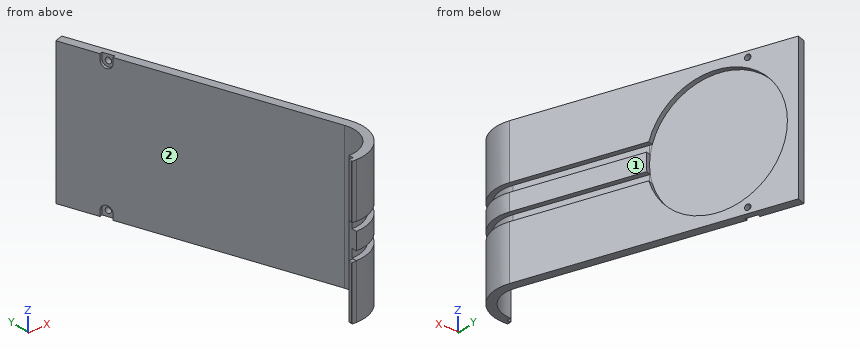
```python
from build123d import *

# Parameters (mm, degrees)
EXTRUDE_1_DEPTH        = 25
SKETCH_4_R             = 22
CUT_EXTRUDE_1_DEPTH    = 1.8
CUT_EXTRUDE_START      = 6
CUT_EXTRUDE_1_2_DEPTH  = 3
SKETCH_11_W            = 18.9
SKETCH_11_H            = 1.4
EXTRUDE_3_DEPTH        = 1.5
FILLET_1_R             = 0.25
SKETCH_12_R            = 1
CUT_EXTRUDE_2553_DEPTH = 99.437390504
CUT_EXTRUDE_1_3_DEPTH  = 1


with BuildPart() as part:
    # 草图2 → 整体拉伸-薄壁1 (new, symmetric)
    with BuildSketch(Plane.XY):
        with BuildLine():
            ThreePointArc((28.874192719, 5.049687275), (37.065713162, 9.313922912), (38.271118927, 18.469888708))
            Line((38.271118927, 18.469888708), (7.496652644, 103.022039918))
            Line((7.496652644, 103.022039918), (10.315730506, 104.048100348))
            Line((10.315730506, 104.048100348), (41.090196789, 19.495949138))
            ThreePointArc((41.090196789, 19.495949138), (39.523169295, 7.593193603), (28.874192719, 2.049687275))
            Line((28.874192719, 2.049687275), (28.874192719, 5.049687275))
        make_face()
    extrude(amount=EXTRUDE_1_DEPTH, both=True)

    # 草图4 → Cut-Extrude 1 (cut)
    with BuildSketch(Plane(origin=(42.549434126, 15.486727507, 0), x_dir=(0, 0, -1), z_dir=(0.9396926207859071, 0.3420201433256726, 0))):
        with Locations(Location((0, 68.845044478, 0), (0, 0, 90))):
            Circle(SKETCH_4_R)
    extrude(amount=-CUT_EXTRUDE_1_DEPTH, mode=Mode.SUBTRACT)

    # 草图3 → Cut-Extrude 1 2 (cut)
    with BuildSketch(Plane.XY.offset(CUT_EXTRUDE_START)):
        with BuildLine():
            ThreePointArc((28.874192719, 3.849687275), (38.048695615, 8.625631188), (39.398750072, 18.88031288))
            Line((39.398750072, 18.88031288), (24.836038582, 58.891033865))
            Line((24.836038582, 58.891033865), (23.809978152, 61.710111727))
            Line((23.809978152, 61.710111727), (25.50142487, 62.325747985))
            Line((25.50142487, 62.325747985), (26.5274853, 59.506670123))
            Line((26.5274853, 59.506670123), (41.090196789, 19.495949138))
            ThreePointArc((41.090196789, 19.495949138), (39.523169295, 7.593193603), (28.874192719, 2.049687275))
            Line((28.874192719, 2.049687275), (28.874192719, 3.849687275))
        make_face()
    cut_extrude_1_2 = extrude(amount=-CUT_EXTRUDE_1_2_DEPTH, mode=Mode.SUBTRACT)

    # 镜向1: Cut-Extrude 1 2 across plane
    add(cut_extrude_1_2.mirror(Plane.XY), mode=Mode.SUBTRACT)

    # 草图11 → 底部卡扣凸台-拉伸3 (add)
    with BuildSketch(Plane.ZY.offset(-28.874192719)):
        with Locations((-15.55, 2.749687275)):
            Rectangle(SKETCH_11_W, SKETCH_11_H)
        with Locations((15.55, 2.749687275)):
            Rectangle(SKETCH_11_W, SKETCH_11_H)
    extrude(amount=EXTRUDE_3_DEPTH)

    # 底部卡扣圆角1
    fillet_1_edges = [part.edges().sort_by_distance(p)[0] for p in [
        (27.374192719, 2.749687275, -25),
        (27.374192719, 2.049687275, -15.55),
        (27.374192719, 2.749687275, -6.1),
        (27.374192719, 3.449687275, -15.55),
        (27.374192719, 2.749687275, 6.1),
        (27.374192719, 2.049687275, 15.55),
        (27.374192719, 2.749687275, 25),
        (27.374192719, 3.449687275, 15.55),
    ]]
    fillet(fillet_1_edges, radius=FILLET_1_R)

    # 草图12 → Cut-Extrude 2553 (cut, through all)
    with BuildSketch(Plane(origin=(39.730356264, 14.460667077, 0), x_dir=(0, 0, 1), z_dir=(-0.9396926207859071, -0.3420201433256726, 0))):
        with Locations(Location((23, 78.482840932, 0), (0, 0, 270))):
            Circle(SKETCH_12_R)
        with Locations(Location((-23, 78.482840932, 0), (0, 0, 270))):
            Circle(SKETCH_12_R)
    extrude(amount=-CUT_EXTRUDE_2553_DEPTH, mode=Mode.SUBTRACT)

    # 草图13 → Cut-Extrude 1 3 (cut)
    with BuildSketch(Plane(origin=(39.730356264, 14.460667077, 0), x_dir=(0, 0, 1), z_dir=(-0.9396926207859071, -0.3420201433256726, 0))):
        with BuildLine():
            Line((23, 80.482840932), (25, 80.482840932))
            Line((25, 80.482840932), (25, 76.482840932))
            Line((25, 76.482840932), (23, 76.482840932))
            ThreePointArc((23, 76.482840932), (21, 78.482840932), (23, 80.482840932))
        make_face()
        with BuildLine():
            Line((-25, 80.482840932), (-25, 76.482840932))
            Line((-25, 76.482840932), (-23, 76.482840932))
            ThreePointArc((-23, 76.482840932), (-21, 78.482840932), (-23, 80.482840932))
            Line((-23, 80.482840932), (-25, 80.482840932))
        make_face()
    extrude(amount=-CUT_EXTRUDE_1_3_DEPTH, mode=Mode.SUBTRACT)


solid = part.part
```
CAD build for the part. Positions are in the model's coordinates, mm. Face numbers are marked on the shaded views. A direction names the side the tool comes from. Coordinates: 2 decimals unless noted, no trailing zeros. Write each loop counter-clockwise with the first axis right and the second up, starting at its lowest first coordinate (ties: lowest second). Pieces come first, ordered by that corner, then holes. Notation, with made-up numbers: (-24.75, 50) -> (26.25, 50) arc R28 ccw to (26.25, 71) -> close; hole circle Ø5 at (0, 72.25). An arc over 180 degrees is marked (long way). Return JSON: item names as keys, results as strings. Group by question number.
Q1. Drill centre lines: line 1 (Z direction, x = 19, y = 80); line 2 (X direction, y = 14.5, z = 7); line 3 (X direction, y = 56, z = 7). Where is each one in solid material? Low to high.
Q2. Cut at C-C, the plane y = 11. Give the cut face in (x, z).
Q3. Which spindle directions (+Z, -Z, +X, -X, +Y, -Y) get a long thin tool onto all of the face, cutting with end or side? Do the marked faces 1 and 2. Say none if no direction does.
Q4. Cut at D-D, the plane z = 13. Give the cut face in (x, y), then the cut area to 3 significant figures.
Q5. Cut at B-B, the plane z = 18.5. Give the cut face in (x, y), then the cut area to 3 significant figures.
Q6. Cut at A-A, the plane x = 32.5. Give the cut face in (y, z).
Q7. Flat gauge pins, fed straight in: pin 1 (1 mm diameter, centred on y = 2.5, z = 18, fed in from -X); pin 2 (5 mm diameter, centred on x = 33, z = -5.5, fed in from -Y); pin 3 (6 mm diameter, centred on y = 68.5, z = -11.5, fed in from +X). Where does each tip first touch, or does it go through?
Returned:
{
 "1": {"line 1": "z = -25 to -22, 22 to 25", "line 2": "x = 38.86 to 41.86", "line 3": "x = 24.61 to 27.8"},
 "2": {"outline": "(38.02, -25) -> (41.23, -25) -> (41.23, -6) -> (39.32, -6) -> (39.32, -3) -> (41.23, -3) -> (41.23, 3) -> (39.32, 3) -> (39.32, 6) -> (41.23, 6) -> (41.23, 25) -> (38.02, 25) -> close"},
 "3": {"face 1": "+Z, -Z, +X, +Y", "face 2": "+Z, -Z, -X"},
 "4": {"outline": "(7.5, 103.02) -> (38.27, 18.47) arc R10 cw to (28.87, 5.05) -> (28.87, 3.45) -> (27.62, 3.45) arc R0.25 ccw to (27.37, 3.2) -> (27.37, 2.3) arc R0.25 ccw to (27.62, 2.05) -> (28.87, 2.05) arc R13 ccw to (41.09, 19.5) -> (25.07, 63.5) -> (23.38, 62.89) -> (11.24, 96.24) -> (12.93, 96.86) -> (10.32, 104.05) -> close", "area": "274 mm2"},
 "5": {"outline": "(7.5, 103.02) -> (38.27, 18.47) arc R10 cw to (28.87, 5.05) -> (28.87, 3.45) -> (27.62, 3.45) arc R0.25 ccw to (27.37, 3.2) -> (27.37, 2.3) arc R0.25 ccw to (27.62, 2.05) -> (28.87, 2.05) arc R13 ccw to (41.09, 19.5) -> (23.08, 68.99) -> (21.38, 68.38) -> (13.24, 90.75) -> (14.93, 91.37) -> (10.32, 104.05) -> close", "area": "295 mm2"},
 "6": {"outline": "(2.57, -25) -> (5.73, -25) -> (5.73, 25) -> (2.57, 25) -> (2.57, 6) -> (4.45, 6) -> (4.45, 3) -> (2.57, 3) -> (2.57, -3) -> (4.45, -3) -> (4.45, -6) -> (2.57, -6) -> close; (34.33, -25) -> (43.1, -25) -> (43.1, -6) -> (37.83, -6) -> (37.83, -3) -> (43.1, -3) -> (43.1, 3) -> (37.83, 3) -> (37.83, 6) -> (43.1, 6) -> (43.1, 25) -> (34.33, 25) -> close"},
 "7": {"pin 1": "stops at x = 27.37", "pin 2": "stops at y = 2.16", "pin 3": "stops at x = 22.43"}
}
